Source: CAD feature listing. Evaluate the final solid. Frame: model axes, mm. A direction names the side the tool comes from. Give positions to 0.01 mm unless a question says otherwise; leave off trailing zeros. Loops run counter-clockwise (first coordinate to the right, second up) from the corner with the lowest first, then second, coordinate; pieces in that order, holes last. Notation, with made-up numbers: M -1.75,70 L 51.25,70 A18 ccw 51.25,98 Z; hole C 9,-30 d8. An arc over 180 degrees is marked long. Answer in a Markdown table with one row per item.
```python
from build123d import *

# Parameters (mm, degrees)
F0_R      = 10
F1_DEPTH  = 20
F1_FACE_R = 10
F2_DEPTH  = 2
F3_W      = 14
F3_H      = 42
F4_DEPTH  = 4


# Not quite as in the source:
# - the program builds the solid bodies; features that only make, move or delete a surface that nothing else refers to are left out


with BuildPart() as f1:
    # F0 (on Front) → F1 (new body)
    with BuildSketch(Plane.XZ):
        with BuildLine():
            Line((45, 25), (-50, 25))
            Line((-50, 25), (-50, -25))
            Line((-50, -25), (45, -25))
            ThreePointArc((45, -25), (48.5355339059, -23.5355339059), (50, -20))
            Line((50, -20), (50, 20))
            ThreePointArc((50, 20), (48.5355339059, 23.5355339059), (45, 25))
        make_face()
        Circle(F0_R, mode=Mode.SUBTRACT)
    extrude(amount=F1_DEPTH)

    # F0 (on Front) + F1_face (on face) → F2 (join)
    with BuildSketch(Plane.XZ):
        with BuildLine():
            Line((45, 25), (-50, 25))
            Line((-50, 25), (-50, -25))
            Line((-50, -25), (45, -25))
            ThreePointArc((45, -25), (48.5355339059, -23.5355339059), (50, -20))
            Line((50, -20), (50, 20))
            ThreePointArc((50, 20), (48.5355339059, 23.5355339059), (45, 25))
        make_face()
        Circle(F0_R, mode=Mode.SUBTRACT)
    with BuildSketch(Plane(origin=(-0.1121943071, -20, 0), x_dir=(1, 0, 0), z_dir=(0, -1, 0))):
        with BuildLine():
            Line((45.1121943071, 25), (-49.8878056929, 25))
            Line((-49.8878056929, 25), (-49.8878056929, -25))
            Line((-49.8878056929, -25), (45.1121943071, -25))
            ThreePointArc((45.1121943071, -25), (48.647728213, -23.5355339059), (50.1121943071, -20))
            Line((50.1121943071, -20), (50.1121943071, 20))
            ThreePointArc((50.1121943071, 20), (48.647728213, 23.5355339059), (45.1121943071, 25))
        make_face()
        with Locations((0.1121943071, 0)):
            Circle(F1_FACE_R, mode=Mode.SUBTRACT)
    extrude(amount=F2_DEPTH)

    # F3 (on face) → F4 (join)
    with BuildSketch(Plane(origin=(-50, 0, 0), x_dir=(0, -1, 0), z_dir=(-1, 0, 0))):
        with Locations((11, 0)):
            Rectangle(F3_W, F3_H)
    extrude(amount=F4_DEPTH)


solid = f1.part
```
Q1. Section query D-D (z = 6.5). Output: boundary loops of the cut face in (x, y).
Values follow:
| item | result |
|---|---|
| outline | M -54,-18 L -50,-18 L -50,-22 L -7.6,-22 L -7.6,0 L -50,0 L -50,-4 L -54,-4 Z; M 7.6,-22 L 50,-22 L 50,0 L 7.6,0 Z |
Q2. Ray query, probe 1 along Z at (x, y) = (0, -8.25); probe 2 along X at (y, z) = (-19, -13); probe 3 along X at (y, z) = (-16.75, 6.5). Return the intervals inside material, ascending. Write a range as from..to.
Values follow:
| item | result |
|---|---|
| probe 1 | -25..-10, 10..25 |
| probe 2 | -50..50 |
| probe 3 | -54..-7.6, 7.6..50 |
Q3. Mould query, pull axis Z, two halves, no side actions, for faces 4 (the flat face through (-3, -11, -25)), 5 (the cylindrical face through (-2.17, -10.85, -9.76)), 6 (the cylindrical face through (49, -11, 23)), 7 (the flat face through (-50, -18.2, 0.3)). Classes: +Z half, -Z half, draft (parallel to the pull), parting line (faces both ways), or undercut.
Values follow:
| item | result |
|---|---|
| face 4 | -Z half |
| face 5 | undercut |
| face 6 | +Z half |
| face 7 | draft |
Q4. Section query C-C (y = -13). Output: boundary loops of the cut face in (x, z).
Values follow:
| item | result |
|---|---|
| outline | M -54,-21 L -50,-21 L -50,-25 L 45,-25 A5 ccw 50,-20 L 50,20 A5 ccw 45,25 L -50,25 L -50,21 L -54,21 Z; hole C 0,0 d20 |
Q5. Reachability of faces 1 (the flat face through (-52, -4, 0)), 2 (the flat face through (-52, -11, 21)), 3 (the flat face through (-52, -11, -21)) from +Z, -Z, +X, -X, +Y, -Y: full face, straight path, thin tool, end or side. Return the list, or none.
Values follow:
| item | result |
|---|---|
| face 1 | +Z, -Z, -X, +Y |
| face 2 | +Z, -X, +Y, -Y |
| face 3 | -Z, -X, +Y, -Y |
Q6. Section query A-A (z = 0). Output: boundary loops of the cut face in (x, y), plus the area to 3 significant figures.
Values follow:
| item | result |
|---|---|
| outline | M -54,-18 L -50,-18 L -50,-22 L -10,-22 L -10,0 L -50,0 L -50,-4 L -54,-4 Z; M 10,-22 L 50,-22 L 50,0 L 10,0 Z |
| area | 1,820 mm^2 |
Q7. Section query B-B (x = 0). Output: boundary loops of the cut face in (y, z).
Values follow:
| item | result |
|---|---|
| outline | M -22,-25 L 0,-25 L 0,-10 L -22,-10 Z; M -22,10 L 0,10 L 0,25 L -22,25 Z |
Q8. Contact query for a flat-ended pin moving along its axis: pin 1 Ø4.5 at (x, z) = (-53, 5.5) entering from +Y. Output: stop coordinate, or through.
Values follow:
| item | result |
|---|---|
| pin 1 | y = -4 |
